```python
from build123d import *

# Parameters (mm, degrees)
BOSS_EXTRUDE1_DEPTH = 6.35
CUT_EXTRUDE1_REACH  = 8.35
SKETCH2_W           = 29.21
SKETCH2_H           = 29.21
FILLET1_R           = 5.08
BOSS_EXTRUDE2_DEPTH = 6.35
FILLET2_R           = 3.81


with BuildPart() as part:
    # Sketch1 → Boss-Extrude1 (new body)
    with BuildSketch(Plane.XY):
        with BuildLine():
            ThreePointArc((-105.206508748, 158.75), (-131.338700922, 79.990592372), (-120.239774453, -2.245346177))
            ThreePointArc((-120.239774453, -2.245346177), (0, -85.336489431), (120.239774453, -2.245346177))
            ThreePointArc((120.239774453, -2.245346177), (131.338700922, 79.990592372), (105.206508748, 158.75))
            ThreePointArc((105.206508748, 158.75), (0, 217.817133941), (-105.206508748, 158.75))
        make_face()
        with BuildLine():
            Line((-101.6, 152.4), (101.6, 152.4))
            ThreePointArc((101.6, 152.4), (125.172151144, 77.635179262), (114.3, 0))
            ThreePointArc((114.3, 0), (0, -78.986489431), (-114.3, 0))
            ThreePointArc((-114.3, 0), (-125.172151144, 77.635179262), (-101.6, 152.4))
        make_face(mode=Mode.SUBTRACT)
    extrude(amount=BOSS_EXTRUDE1_DEPTH)

    # Sketch2 → Cut-Extrude1 (cut, up to next)
    with BuildSketch(Plane.XY.offset(6.35), mode=Mode.PRIVATE) as cut_extrude1_sk1:
        with Locations((0, 185.10856697)):
            Rectangle(SKETCH2_W, SKETCH2_H)
    cut_extrude1_tool1 = extrude(cut_extrude1_sk1.sketch, amount=-CUT_EXTRUDE1_REACH, mode=Mode.PRIVATE) & part.part
    add(cut_extrude1_tool1.solids().sort_by_distance((0, 185.108567, 6.35))[0], mode=Mode.SUBTRACT)

    # Fillet1
    fillet1_edges = [part.edges().sort_by_distance(p)[0] for p in [
        (14.605, 199.71356697, 3.175),
        (14.605, 170.50356697, 3.175),
        (-14.605, 170.50356697, 3.175),
        (-14.605, 199.71356697, 3.175),
    ]]
    fillet(fillet1_edges, radius=FILLET1_R)

    # Sketch3 → Boss-Extrude2 (add)
    with BuildSketch(Plane.XY.offset(6.35)):
        Polygon((-100.252961582, 153.747038418), (-102.947038418, 151.052961582), (-2.694076836, 50.8), (-93.720570633, -40.226493797), (-91.026493797, -42.920570633), (0, 48.105923164), (91.026493797, -42.920570633), (93.720570633, -40.226493797), (2.694076836, 50.8), (102.947038418, 151.052961582), (100.252961582, 153.747038418), (0, 53.494076836), align=None)
    extrude(amount=-BOSS_EXTRUDE2_DEPTH)

    # Fillet2
    fillet2_edges = [part.edges().sort_by_distance(p)[0] for p in [
        (102.584006308, 150.689929472, 3.175),
        (98.905923164, 152.4, 3.175),
        (-88.818700326, -40.712777162, 3.175),
        (-91.394282222, -37.900205386, 3.175),
        (0, 53.494076836, 3.175),
        (-102.584006308, 150.689929472, 3.175),
        (-98.905923164, 152.4, 3.175),
        (0, 48.105923164, 3.175),
        (88.818700326, -40.712777162, 3.175),
        (91.394282222, -37.900205386, 3.175),
        (2.694076836, 50.8, 3.175),
        (-2.694076836, 50.8, 3.175),
    ]]
    fillet(fillet2_edges, radius=FILLET2_R)


solid = part.part
```
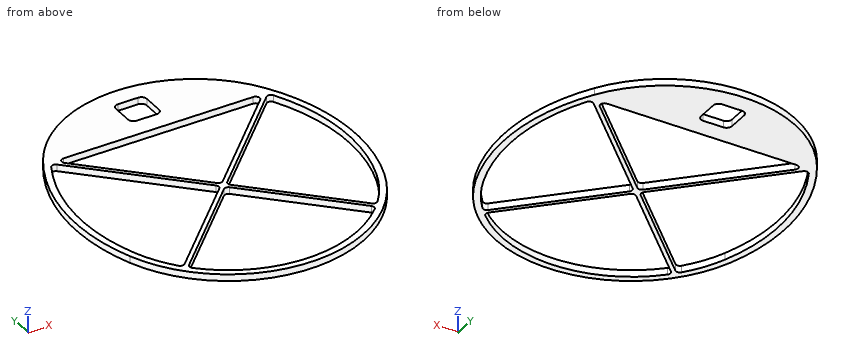
Source: CAD feature listing. Evaluate the final solid. Frame: model axes, mm. Coordinates: 2 decimals unless noted, no trailing zeros. Order: outer loops, then holes, each group sorted by start corner. A loop starts at its lowest first (then second) coordinate and runs counter-clockwise, first axis right, second up. Notation, with made-up numbers: (-34, -1.75) - (17, -1.75) arc R10 ccw to (17, 13.25) - close; hole circle Ø5 at (25, -22). An arc over 180 degrees is marked (long way). One line per item, written item: value.
1) Cut plane B-B on x = 67.5. Output: boundary loops of the cut face in (y, z).
Computed values:
outline: (-66.19, 0) - (-58.65, 0) - (-58.65, 6.35) - (-66.19, 6.35) - close; (-19.39, 0) - (-14.01, 0) - (-14.01, 6.35) - (-19.39, 6.35) - close; (115.61, 0) - (120.99, 0) - (120.99, 6.35) - (115.61, 6.35) - close; (152.4, 0) - (197.69, 0) - (197.69, 6.35) - (152.4, 6.35) - close
2) Cut plane C-C on y = -50. Output: boundary loops of the cut face in (x, z).
Computed values:
outline: (-88.52, 0) - (-79.02, 0) - (-79.02, 6.35) - (-88.52, 6.35) - close; (79.02, 0) - (88.52, 0) - (88.52, 6.35) - (79.02, 6.35) - close
3) Ray query, line 1 (Y direction, x = -22, z = 0.5); line 2 (Y direction, x = 47, z = 5.5); line 3 (Y direction, x = -91.5, z = 5.5). Return the intervals inside material, ascending. Write a range as [from, to].
Computed values:
line 1: y = [-83.44, -76.99], [26.11, 31.49], [70.11, 75.49], [152.4, 215.84]
line 2: y = [-76.44, -69.59], [1.11, 6.49], [95.11, 100.49], [152.4, 208.5]
line 3: y = [-47.08, -36.09], [139.61, 144.99], [151.95, 177.13]
4) Cut plane A-A on y = 106.5. Output: boundary loops of the cut face in (x, z).
Computed values:
outline: (-126.89, 0) - (-120.35, 0) - (-120.35, 6.35) - (-126.89, 6.35) - close; (-58.39, 0) - (-53.01, 0) - (-53.01, 6.35) - (-58.39, 6.35) - close; (53.01, 0) - (58.39, 0) - (58.39, 6.35) - (53.01, 6.35) - close; (120.35, 0) - (126.89, 0) - (126.89, 6.35) - (120.35, 6.35) - close
5) Contact query for flat-ended pins moving along their axis: pin 1 (3 mm diameter, centred on y = 182.5, z = 2, fed in from -X); pin 2 (3 mm diameter, centred on y = 183.5, z = 2, fed in from +X). Output: stop coordinate, or through.
Computed values:
pin 1: stops at x = -87.85
pin 2: stops at x = 86.86
6) Cut plane D-D on z = 1.5. State how many separate pieces and enclosed holes the cut face has, plus the area to 3 significant figures.
Computed values:
separate pieces: 1
enclosed holes: 5
area: 15,400 mm^2
